Input: dimensioned drawing with shaded views. Units: mm. Origin: part minimum x, y, z. A direction names the side the tool comes from. Coordinates: 2 decimals unless noted, no trailing zeros. Order: outer loops, then holes, each group sorted by start corner. A loop starts at its lowest first (then second) coordinate and runs counter-clockwise, first axis right, second up. Notation, with made-up numbers: (-21.5, 34) -> (14.5, 34) arc R16 cw to (14.5, 51) -> close; hole circle Ø9 at (-38, 63.5). An arc over 180 degrees is marked (long way). Answer in a Markdown table with one row per item. Add a question column.
1) Section query C-C on y = 14.25. Return the cut outline in (x, z).
2) Ray query, line 1 (Z direction, x = 21.5, y = 11.25); line 2 (Y direction, x = 18, z = 13); line 3 (X direction, y = 4.5, z = 9). Return the intervals inside material, ascending. Write a range as from..to.
3) Contact query for flat-ended pins moving along their axis: P1, Ø10, axis at y = 9.5, z = 31.5, coming from the +X side; P2, Ø10, axis at x = 8, y = 12.5, coming from the -Z side; P3, Ø8, axis at x = 35.5, y = 9.5, coming from the +Z side. Output: stop coordinate, or through.
4) Set-up query: the marked faces 1 and 2. Return all of +Z, -Z, +X, -X, +Y, -Y with unobstructed straight access to the full face (end or side cutting, diameter ignored); none if empty.
5) Section query D-D on y = 1.5. Return the cut outline in (x, z) (1 decimal), then the cut area to 3 significant figures.
6) Section query B-B on z = 21.5. Return the cut outline in (x, y).
7) Pull-direction query (X, two-part tool) for the marked faces 3, 4 and 5; classes: +X half, -X half, draft (parallel to the pull), parting line (faces both ways), or undercut.
8) Section query A-A on x = 21.5. Return the cut outline in (y, z).
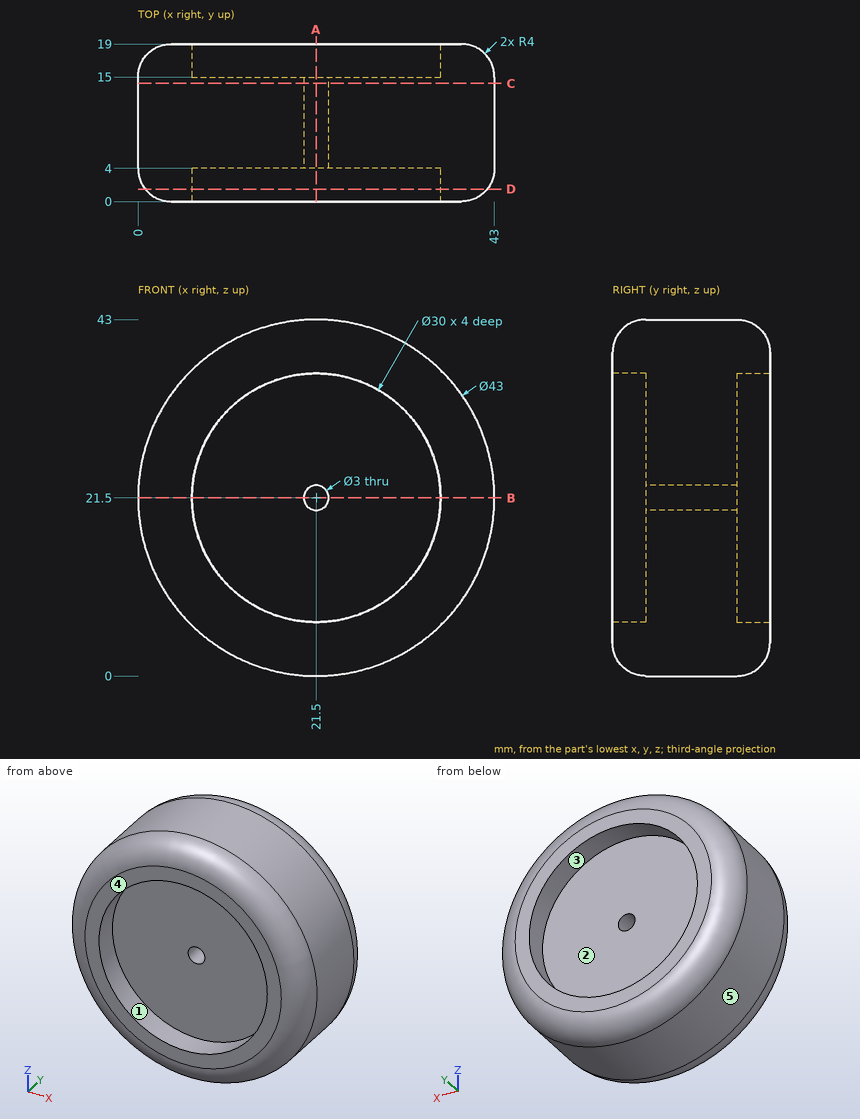
Result:
| question | item | result |
|---|---|---|
| 1 | outline | circle Ø43 at (21.5, 21.5); hole circle Ø3 at (21.5, 21.5) |
| 2 | line 1 | 0..20, 23..43 |
| 2 | line 2 | 4..15 |
| 2 | line 3 | 4.01..38.99 |
| 3 | P1 | x = 42.41 |
| 3 | P2 | z = 1.75 |
| 3 | P3 | z = 40.53 |
| 4 | face 1 | -Y |
| 4 | face 2 | +Y |
| 5 | outline | circle Ø41.2 at (21.5, 21.5); hole circle Ø30 at (21.5, 21.5) |
| 5 | area | 629 mm2 |
| 6 | outline | (0, 4) arc R4 ccw to (4, 0) -> (6.5, 0) -> (6.5, 4) -> (20, 4) -> (20, 15) -> (6.5, 15) -> (6.5, 19) -> (4, 19) arc R4 ccw to (0, 15) -> close; (23, 4) -> (36.5, 4) -> (36.5, 0) -> (39, 0) arc R4 ccw to (43, 4) -> (43, 15) arc R4 ccw to (39, 19) -> (36.5, 19) -> (36.5, 15) -> (23, 15) -> close |
| 7 | face 3 | undercut |
| 7 | face 4 | draft |
| 7 | face 5 | parting line |
| 8 | outline | (0, 4) arc R4 ccw to (4, 0) -> (15, 0) arc R4 ccw to (19, 4) -> (19, 6.5) -> (15, 6.5) -> (15, 20) -> (4, 20) -> (4, 6.5) -> (0, 6.5) -> close; (0, 36.5) -> (4, 36.5) -> (4, 23) -> (15, 23) -> (15, 36.5) -> (19, 36.5) -> (19, 39) arc R4 ccw to (15, 43) -> (4, 43) arc R4 ccw to (0, 39) -> close |
